Part model, mm, in its own coordinate system. Face numbers are marked on the shaded views. A direction names the side the tool comes from. Coordinates: 2 decimals unless noted, no trailing zeros. Write each loop counter-clockwise with the first axis right and the second up, starting at its lowest first coordinate (ties: lowest second). Pieces come first, ordered by that corner, then holes. Notation, with made-up numbers: (31.25, 40) -> (52.25, 40) arc R35 ccw to (52.25, 79) -> close; hole circle Ø8 at (11, 69). An arc over 180 degrees is marked (long way). One line per question, with ' | ' between items. Start each with the question number.
Item 1: Pin check, flat tips, straight feed: pin 1 (4 mm diameter, centred on x = 0.5, y = -28.5, fed in from +Z); pin 2 (3.5 mm diameter, centred on y = 32.5, z = 30.5, fed in from -X); pin 3 (8 mm diameter, centred on x = -19.5, z = 34, fed in from +Y); pin 4 (2 mm diameter, centred on y = 14, z = 39.5, fed in from +X). Stop position of each tip, or through.
Item 2: Saw through at D-D (y = 21). List the corners of the cut face in (x, z), and give its area (3 significant figures).
Item 3: Two-plate mould, pull along Y, no slides. Class the marked faces 4, 5 and 6: pulls with the +Y half, pulls with the -Y half, needs draft (parallel to the pull), parting line crosses it, or undercut.
Item 4: Saw through at B-B (y = -29.21). List the corners of the cut face in (x, z) (3 decimals), and give its area (3 significant figures).
Item 5: Saw through at A-A (z = 37). List the corners of the cut face in (x, y) (3 decimals).
Item 6: 3-axis set-ups, long thin cutter, end or side, ignore diameter. For the marked faces 1, 2 and 3: which of +Z, -Z, +X, -X, +Y, -Y reach the whole face in a straight line?
Item 7: Saw through at C-C (x = 0). List the corners of the cut face in (y, z).
Item 8: Probe probe 1 along Y at (x, z) = (-5, 35.5); probe 2 along X at (y, z) = (-1.5, 34) (3 decimals); probe 3 along Z at (x, y) = (-16.5, -15). List the from-to ranges inside material, lowest first. Write a range as [from, to].
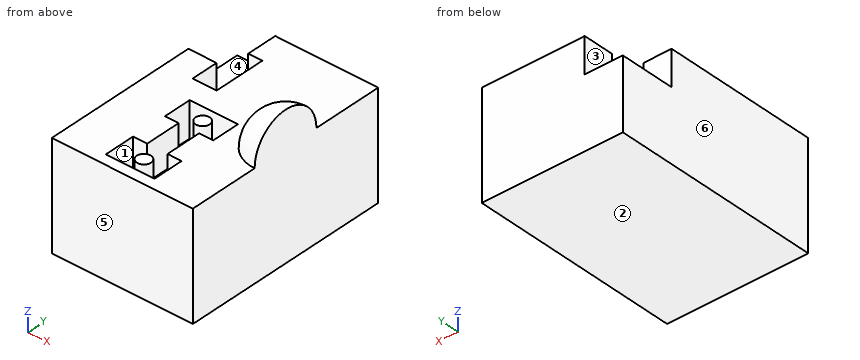
from build123d import *

# Parameters (mm, degrees)
F0_W     = 50.8
F0_H     = 76.2
F1_DEPTH = 38.1
F3_ANGLE = 90
F4_DEPTH = 12.7
F2_R     = 2.54
F5_DEPTH = 12.7


with BuildPart() as f1:
    # F0 (on Top) → F1 (new body)
    with BuildSketch(Plane.XY):
        Rectangle(F0_W, F0_H)
    extrude(amount=F1_DEPTH)

    # F2 (on face) → F3 (revolve)
    with BuildSketch(Plane.XY.offset(38.1)):
        with BuildLine():
            Line((25.4, -12.7), (25.4, 12.7))
            ThreePointArc((25.4, 12.7), (12.7, 0), (25.4, -12.7))
        make_face()
    revolve(axis=Axis((25.4, 0, 38.1), (0, 1, 0)), revolution_arc=F3_ANGLE)

    # F2 (on face) → F4 (cut)
    with BuildSketch(Plane.XY.offset(38.1)):
        Polygon((-11.684, 38.1), (-25.4, 38.1), (-25.4, 18.034), (-15.24, 18.034), (-15.24, 8.1802008182), (-6.604, 8.1802008182), (-6.604, 26.9762008182), (-11.684, 26.9762008182), align=None)
    extrude(amount=-F4_DEPTH, mode=Mode.SUBTRACT)

    # F2 (on face) → F5 (cut)
    with BuildSketch(Plane.XY.offset(38.1)):
        Polygon((-9.271, -23.114), (-9.271, -34.29), (8.255, -34.29), (8.255, -23.114), (3.175, -23.114), (3.175, -10.16), (8.255, -10.16), (8.255, 0), (-9.1186, 0), (-9.1186, -10.16), (-4.191, -10.16), (-4.191, -23.114), align=None)
        with Locations((0, -29.21)):
            Circle(F2_R, mode=Mode.SUBTRACT)
        with Locations((0, -5.08)):
            Circle(F2_R, mode=Mode.SUBTRACT)
    extrude(amount=-F5_DEPTH, mode=Mode.SUBTRACT)


solid = f1.part
From the geometry:
1) pin 1: z = 38.1 | pin 2: x = -11.68 | pin 3: y = 18.03 | pin 4: through
2) outline: (-25.4, 0) -> (25.4, 0) -> (25.4, 38.1) -> (-6.6, 38.1) -> (-6.6, 25.4) -> (-25.4, 25.4) -> close | area: 1,700 mm2
3) face 4: undercut | face 5: pulls with the -Y half | face 6: needs draft
4) outline: (-25.4, 0) -> (25.4, 0) -> (25.4, 38.1) -> (8.255, 38.1) -> (8.255, 25.4) -> (2.54, 25.4) -> (2.54, 38.1) -> (-2.54, 38.1) -> (-2.54, 25.4) -> (-9.271, 25.4) -> (-9.271, 38.1) -> (-25.4, 38.1) -> close | area: 1,780 mm2
5) outline: (-25.4, -38.1) -> (25.4, -38.1) -> (25.4, 38.1) -> (-11.684, 38.1) -> (-11.684, 26.976) -> (-6.604, 26.976) -> (-6.604, 8.18) -> (-15.24, 8.18) -> (-15.24, 18.034) -> (-25.4, 18.034) -> close; circle Ø5.08 at (0, -29.21); circle Ø5.08 at (0, -5.08); hole (-9.271, -34.29) -> (8.255, -34.29) -> (8.255, -23.114) -> (3.175, -23.114) -> (3.175, -10.16) -> (8.255, -10.16) -> (8.255, 0) -> (-9.119, 0) -> (-9.119, -10.16) -> (-4.191, -10.16) -> (-4.191, -23.114) -> (-9.271, -23.114) -> close
6) face 1: +Z | face 2: -Z, +X, -X, +Y, -Y | face 3: +Z, -X, +Y
7) outline: (-38.1, 0) -> (38.1, 0) -> (38.1, 38.1) -> (0, 38.1) -> (0, 25.4) -> (-2.54, 25.4) -> (-2.54, 38.1) -> (-7.62, 38.1) -> (-7.62, 25.4) -> (-26.67, 25.4) -> (-26.67, 38.1) -> (-31.75, 38.1) -> (-31.75, 25.4) -> (-34.29, 25.4) -> (-34.29, 38.1) -> (-38.1, 38.1) -> close
8) probe 1: [-38.1, -34.29], [-23.11, -10.16], [0, 38.1] | probe 2: [-25.4, -9.119], [8.255, 25.4] | probe 3: [0, 38.1]
